```python
from build123d import *

# Parameters (mm, degrees)
SKETCH1_W           = 112.384257698
SKETCH1_H           = 69.188872884
BOSS_EXTRUDE1_DEPTH = 12
CHAMFER3_SIZE       = 12
CHAMFER4_SIZE       = 12


with BuildPart() as part:
    # Sketch1 → Boss-Extrude1 (new body)
    with BuildSketch(Plane(origin=(0, 0, 0), x_dir=(1, 0, 0), z_dir=(0, 1, 0))):
        Rectangle(SKETCH1_W, SKETCH1_H)
    extrude(amount=BOSS_EXTRUDE1_DEPTH)

    # Chamfer3
    chamfer3_edges = [part.edges().sort_by_distance(p)[0] for p in [
        (56.192128849, 6, 34.594436442),
    ]]
    chamfer(chamfer3_edges, length=CHAMFER3_SIZE)

    # Chamfer4
    chamfer4_edges = [part.edges().sort_by_distance(p)[0] for p in [
        (56.192128849, 6, -34.594436442),
    ]]
    chamfer(chamfer4_edges, length=CHAMFER4_SIZE)


solid = part.part
```
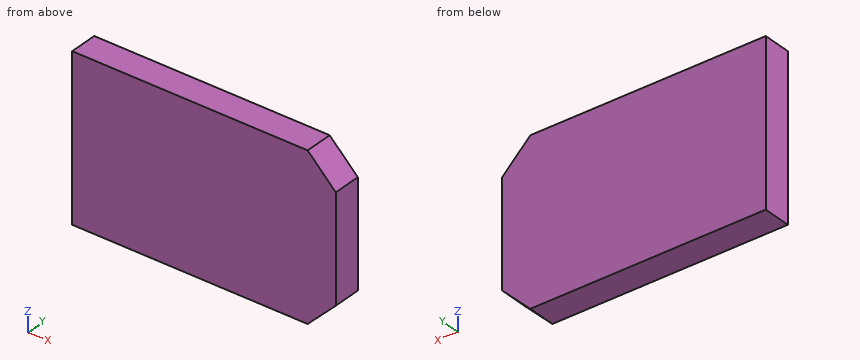
Work out the finished part from the listing and answer in its coordinate system (mm). Round coordinates to 2 decimals unless told otherwise and drop trailing zeros. Write each loop counter-clockwise with the first axis right and the second up, starting at its lowest first coordinate (ties: lowest second). Pieces come first, ordered by that corner, then holes.
1) Consider probe 1 along X at (y, z) = (3.25, -25); probe 2 along X at (y, z) = (7.5, 23). Determine where each line is inside the solid, lowest interval first.
2) A cutting plane is placed at B-B on x = 46.5. Determine the outline of the cut face in (y, z), and give its area (3 significant figures).
3) A cutting plane is placed at C-C on z = 26. Determine the outline of the cut face in (x, y).
4) A flat-ended cylindrical pin translates along its axis: P1, Ø6, axis at x = -45, z = -10.5, coming from the -Y side. Find the tip coordinate at first contact, or state that the pin passes through.
5) A cutting plane is placed at A-A on y = 5.25. Determine the outline of the cut face in (x, z).
Entries:
1. probe 1: x = -56.19 to 53.79
1. probe 2: x = -56.19 to 55.79
2. outline: (0, -32.29) - (12, -32.29) - (12, 32.29) - (0, 32.29) - close
2. area: 775 mm2
3. outline: (-56.19, 0) - (52.79, 0) - (52.79, 12) - (-56.19, 12) - close
4. P1: stops at y = 0
5. outline: (-56.19, -34.59) - (44.19, -34.59) - (56.19, -22.59) - (56.19, 22.59) - (44.19, 34.59) - (-56.19, 34.59) - close
